For this review, take the finished solid that the model builds, in its own axes (mm). A direction names the side the tool comes from. Coordinates: 2 decimals unless noted, no trailing zeros. Loops run counter-clockwise (first coordinate to the right, second up) from the corner with the lowest first, then second, coordinate; pieces in that order, holes last. Notation, with made-up numbers: M 74,80 L 104,80 A24 cw 104,112 Z; hole C 57,62 d9. An arc over 180 degrees is marked long. Write each question's results on one line, items separated by ' | '. Start each with the question number.
```python
from build123d import *

# Parameters (mm, degrees)
SKETCH1_R           = 0.9
SKETCH1_R_2         = 1.4
BOSS_EXTRUDE1_DEPTH = 3.175
FILLET1_R           = 1


with BuildPart() as part:
    # Sketch1 → Boss-Extrude1 (new body)
    with BuildSketch(Plane.XY):
        Polygon((31.690894529, -38.1), (31.690894529, 0), (20, 0), (20, 10.87553853), (0, 10.87553853), (0, 0), (-6.409105471, 0), (-6.409105471, -38.1), align=None)
        with Locations((26.490894529, -32.9)):
            Circle(SKETCH1_R, mode=Mode.SUBTRACT)
        with Locations((-1.209105471, -32.9)):
            Circle(SKETCH1_R, mode=Mode.SUBTRACT)
        with Locations((-1.209105471, -5.2)):
            Circle(SKETCH1_R, mode=Mode.SUBTRACT)
        with Locations((26.490894529, -5.2)):
            Circle(SKETCH1_R, mode=Mode.SUBTRACT)
        with Locations((16.335044769, 3.811593223)):
            Circle(SKETCH1_R_2, mode=Mode.SUBTRACT)
        with Locations((3.664955231, 3.811593223)):
            Circle(SKETCH1_R_2, mode=Mode.SUBTRACT)
        with BuildLine():
            Line((26.490894529, -7.1), (26.490894529, -31))
            ThreePointArc((26.490894529, -31), (25.147391645, -31.556497116), (24.590894529, -32.9))
            Line((24.590894529, -32.9), (0.690894529, -32.9))
            ThreePointArc((0.690894529, -32.9), (0.134397413, -31.556497116), (-1.209105471, -31))
            Line((-1.209105471, -31), (-1.209105471, -7.1))
            ThreePointArc((-1.209105471, -7.1), (0.134397413, -6.543502884), (0.690894529, -5.2))
            Line((0.690894529, -5.2), (24.590894529, -5.2))
            ThreePointArc((24.590894529, -5.2), (25.147391645, -6.543502884), (26.490894529, -7.1))
        make_face(mode=Mode.SUBTRACT)
    extrude(amount=BOSS_EXTRUDE1_DEPTH)

    # Fillet1
    fillet1_edges = [part.edges().sort_by_distance(p)[0] for p in [
        (20, 10.87553853, 1.5875),
        (20, 0, 1.5875),
        (31.690894529, 0, 1.5875),
        (31.690894529, -38.1, 1.5875),
        (-6.409105471, -38.1, 1.5875),
        (-6.409105471, 0, 1.5875),
        (0, 0, 1.5875),
        (0, 10.87553853, 1.5875),
    ]]
    fillet(fillet1_edges, radius=FILLET1_R)


solid = part.part
```
Q1. For faces 5 (the face through (20, 5, 2)), 6 (the face through (25.133, -6.529, 1.565)), 7 (the face through (0, 5, 2)), list the 3-axis set-ups (+Z, -Z, +X, -X, +Y, -Y) from which the entire face can be reached by the end or side of a thin tool; tool diameter is ignored.
Q2. To check wall thickness, follow line 1 along Y through (x, z) = (16.5, 2.35); line 2 along X through (y, z) = (-33, 0.7); line 3 along Y through (x, z) = (24.5, 2.2). State the ranges of each line that lie inside material, in increasing order.
Q3. Insertion check: P1, Ø1.1, axis at x = 26.49, y = -32.9, coming from the -Z side; P2, Ø1, axis at y = 5.5, z = 1.5, coming from the +X side; P3, Ø1.6, axis at x = 28, z = 1.5, coming from the +Y side. Each pin has a flat end and moves straight along its axis. Give the tip position at first contact, or say it passes through.
Q4. Take a section at D-D, the plane z = 0.9. Give the number of separate pieces and of enclosed holes in the cut face, then the cut area to 3 significant figures.
Q5. Take a section at A-A, the plane x = 14. Give the boundary of the cut face in (y, z) (3 decimals).
Q6. The part is to be moulded in two halves that separate along X. For faces 1 (the face through (12, -5.2, 2)), 2 (the face through (12, -38.1, 2)), 3 (the face through (20.301, 0.285, 1.61)), 4 (the face through (13, -32.9, 2)), say which applies: pulls with the +X half, pulls with the -X half, needs draft (parallel to the pull), parting line crosses it, or undercut.
Q7. Take a section at C-C, the plane x = 4. Give the boundary of the cut face in (y, z) (3 decimals), then the cut area to 3 significant figures.
Q8. Take a section at B-B, the plane y = -27. Give the boundary of the cut face in (x, z) (3 decimals).
Results:
1) face 5: +Z, -Z, +X, +Y | face 6: +Z, -Z | face 7: +Z, -Z, -X, +Y
2) line 1: -38.1 to -32.9, -5.2 to 2.42, 5.2 to 10.88 | line 2: -6.41 to -2.1, -0.31 to 25.6, 27.39 to 31.69 | line 3: -38.1 to -32.9, -5.2 to 0
3) P1: through | P2: x = 20 | P3: y = 0
4) separate pieces: 1 | enclosed holes: 7 | area: 890 mm^2
5) outline: M -38.1,0 L -32.9,0 L -32.9,3.175 L -38.1,3.175 Z; M -5.2,0 L 10.876,0 L 10.876,3.175 L -5.2,3.175 Z
6) face 1: undercut | face 2: needs draft | face 3: pulls with the +X half | face 4: undercut
7) outline: M -38.1,0 L -32.9,0 L -32.9,3.175 L -38.1,3.175 Z; M -5.2,0 L 2.452,0 L 2.452,3.175 L -5.2,3.175 Z; M 5.171,0 L 10.876,0 L 10.876,3.175 L 5.171,3.175 Z | area: 58.9 mm^2
8) outline: M -6.409,0 L -1.209,0 L -1.209,3.175 L -6.409,3.175 Z; M 26.491,0 L 31.691,0 L 31.691,3.175 L 26.491,3.175 Z
